Source: CAD feature listing. Evaluate the final solid. Frame: model axes, mm. Give positions to 0.01 mm unless a question says otherwise; leave off trailing zeros. Order: outer loops, then holes, each group sorted by start corner. A loop starts at its lowest first (then second) coordinate and runs counter-clockwise, first axis right, second up. Notation, with made-up numbers: M 28.5,6 L 53.5,6 A26 ccw 53.5,25 Z; hole C 80.5,-7 d4. An arc over 180 degrees is marked long. Answer as a JSON object with one key per item and string values. Group by question number.
1. Pin query (flat end, axial travel): P1, Ø1.5, axis at y = -1.5, z = 1.5, coming from the +X side; P2, Ø2, axis at x = -15, y = 0, coming from the -Z side. Return the tip coordinate at first contact, or that it passes through.
2. Pull-direction query (Y, two-part tool) for faces 1 (the cylindrical face through (17.674, 0.059, 0.031)), 2 (the flat face through (0, -2, 2.25)), 3 (the cylindrical face through (-13.4, 0.5, 0)); classes: +Y half, -Y half, draft (parallel to the pull), parting line (faces both ways), or undercut.
3. Section query B-B (x = 0). Output: boundary loops of the cut face in (y, z) (3 decimals), plus the area to 3 significant figures.
4. Section query C-C (z = -0.25). Output: boundary loops of the cut face in (x, y) (3 decimals).
5. Section query D-D (y = -2.1). Output: boundary loops of the cut face in (x, z), plus the area to 3 significant figures.
6. Material intervals for L1, parallel to Y at x = 0, z = -0.9 (3 decimals); L2, parallel to X at y = 0.25, z = -2; L3, parallel to X at y = 0.75, z = -1.7, sorted ascending. Write a range as [from, to].
7. Section query A-A (y = 0). Output: boundary loops of the cut face in (x, z) (3 decimals).
from build123d import *

# Parameters (mm, degrees)
SKETCH1_R           = 1.675
BOSS_EXTRUDE1_DEPTH = 2.25


with BuildPart() as part:
    # Sketch1 → Boss-Extrude1 (new body, symmetric)
    with BuildSketch(Plane.XY):
        with BuildLine():
            Line((-15, 2.675), (15, 2.675))
            ThreePointArc((15, 2.675), (17.675, 0), (15, -2.675))
            Line((15, -2.675), (-15, -2.675))
            ThreePointArc((-15, -2.675), (-17.675, 0), (-15, 2.675))
        make_face()
        with Locations((-15, 0)):
            Circle(SKETCH1_R, mode=Mode.SUBTRACT)
        with Locations((-7.5, 0)):
            Circle(SKETCH1_R, mode=Mode.SUBTRACT)
        Circle(SKETCH1_R, mode=Mode.SUBTRACT)
        with Locations((7.5, 0)):
            Circle(SKETCH1_R, mode=Mode.SUBTRACT)
        with Locations((15, 0)):
            Circle(SKETCH1_R, mode=Mode.SUBTRACT)
    extrude(amount=BOSS_EXTRUDE1_DEPTH, both=True)


solid = part.part
Answer sheet:
{
 "1": {"P1": "x = 17.57", "P2": "through"},
 "2": {"face 1": "parting line", "face 2": "draft", "face 3": "undercut"},
 "3": {"outline": "M -2.675,-2.25 L -1.675,-2.25 L -1.675,2.25 L -2.675,2.25 Z; M 1.675,-2.25 L 2.675,-2.25 L 2.675,2.25 L 1.675,2.25 Z", "area": "9.00 mm^2"},
 "4": {"outline": "M -15,-2.675 L 15,-2.675 A2.675 ccw 15,2.675 L -15,2.675 A2.675 ccw Z; hole C -15,0 d3.35; hole C -7.5,0 d3.35; hole C 0,0 d3.35; hole C 7.5,0 d3.35; hole C 15,0 d3.35"},
 "5": {"outline": "M -16.66,-2.25 L 16.66,-2.25 L 16.66,2.25 L -16.66,2.25 Z", "area": "150 mm^2"},
 "6": {"L1": "[-2.675, -1.675], [1.675, 2.675]", "L2": "[-17.66, -16.66], [-13.34, -9.16], [-5.84, -1.66], [1.66, 5.84], [9.16, 13.34], [16.66, 17.66]", "L3": "[-17.57, -16.5], [-13.5, -9], [-6, -1.5], [1.5, 6], [9, 13.5], [16.5, 17.57]"},
 "7": {"outline": "M -17.675,-2.25 L -16.675,-2.25 L -16.675,2.25 L -17.675,2.25 Z; M -13.325,-2.25 L -9.175,-2.25 L -9.175,2.25 L -13.325,2.25 Z; M -5.825,-2.25 L -1.675,-2.25 L -1.675,2.25 L -5.825,2.25 Z; M 1.675,-2.25 L 5.825,-2.25 L 5.825,2.25 L 1.675,2.25 Z; M 9.175,-2.25 L 13.325,-2.25 L 13.325,2.25 L 9.175,2.25 Z; M 16.675,-2.25 L 17.675,-2.25 L 17.675,2.25 L 16.675,2.25 Z"}
}
